Read the model definition and answer for the solid it produces. Units are mm, in the model's axes. Face numbers are marked on the shaded views. Coordinates: 2 decimals unless noted, no trailing zeros. Loops run counter-clockwise (first coordinate to the right, second up) from the corner with the lowest first, then second, coordinate; pieces in that order, holes last. Notation, with made-up numbers: M 45.5,-4.75 L 68.5,-4.75 A35 ccw 68.5,28.25 Z; hole C 41,28.5 d3. An arc over 180 degrees is marked long. One line per item, written item: value. Start each with the question number.
1. The part is cut by section A-A (x = 10). Write down the section's boundary in (y, z), then the cut area to 3 significant figures.
2. Determine the mould class of the marked faces 1, 2, 3 and 4 for opening direction X: +X half, -X half, draft (parallel to the pull), parting line (faces both ways), or undercut.
3. Flat-ended cylindrical pins translate along their axes: pin 1 (3 mm diameter, centred on x = 0, y = -2, fed in from -Z); pin 2 (5 mm diameter, centred on y = 6, z = 1.5, fed in from +X); pin 3 (5 mm diameter, centred on y = -5, z = 1.5, fed in from -X); pin 4 (4.5 mm diameter, centred on x = 10, y = 10, fed in from -Z). Find the tip coordinate at first contact, or state that the pin passes through.
4. Consider probe 1 along X at (y, z) = (10, 9.05); probe 2 along Y at (x, z) = (10, 4.75); probe 3 along Y at (x, z) = (-10, 9.2). Determine where each line is inside the solid, lowest interval first.
5. The part is cut by section B-B (z = 5.5). Write down the section's boundary in (x, y), then the cut area to 3 significant figures.
6. The part is cut by section D-D (y = -2.5). Write down the section's boundary in (x, z), then the cut area to 3 significant figures.
Autodesk Fusion 360 part; units mm, degrees
sketch "Sketch1" plane through (0, 0, 0) normal (0, 0, 1) x (1, 0, 0)
  line L0 (20, -20) -> (-20, -20)
  line L1 (-20, -20) -> (-20, 20)
  line L2 (-20, 20) -> (20, 20)
  line L3 (20, 20) -> (20, -20)
  line L4 (20, -20) -> (-20, 20) construction
  line L5 (-20, -20) -> (20, 20) construction
  dimension "d1" = 40
  dimension "d2" = 40
extrude "Extrude1" add sketch "Sketch1" along normal blind 5
chamfer "Chamfer1" distance 8 angle 30 4 edges at (20, 0, 0) (0, -20, 0) (-20, 0, 0) (0, 20, 0) measured on face at (6.6667, -6.6667, 0) measured on face at (6.6667, -6.6667, 0) measured on face at (6.6667, -6.6667, 0) measured on face at (6.6667, -6.6667, 0)
extrude "Extrude2" add 1 faces at (6.6667, -6.6667, 5) along direction (0, 0, 1) blind 5
sketch "Sketch2" plane through (0, 0, 10) normal (0, 0, 1) x (-1, 0, 0)
  line L0 (-20, -20) -> (20, -20)
  line L1 (20, -20) -> (20, 20)
  line L2 (20, 20) -> (-20, 20)
  line L3 (-20, 20) -> (-20, -20)
  circle A0 centre (10, 10) radius 2.5
  circle A1 centre (-10, -10) radius 2.5
  circle A2 centre (10, 10) radius 4.5
  circle A3 centre (-10, -10) radius 4.5
  dimension "d11" = 5
  dimension "d12" = 5
  dimension "d15" = 9
  dimension "d16" = 9
  dimension "d20" = 10
  dimension "d21" = 10
  dimension "d22" = 10
  dimension "d23" = 10
extrude "Extrude4" cut sketch "Sketch2" along normal blind 7 from surface at -10 contours A2 | A3
extrude "Extrude3" cut sketch "Sketch2" against normal up to surface (10 mm away) contours A0 | A1
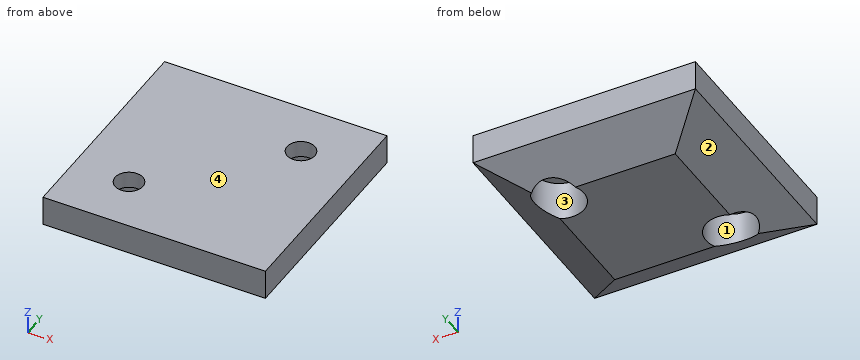
Answer block:
1. outline: M -20,4.62 L -12,0 L 5.5,0 L 5.5,7 L 7.5,7 L 7.5,10 L -20,10 Z; M 12.5,7 L 14.5,7 L 14.5,1.44 L 20,4.62 L 20,10 L 12.5,10 Z
1. area: 287 mm2
2. face 1: undercut
2. face 2: -X half
2. face 3: undercut
2. face 4: draft
3. pin 1: stops at z = 0
3. pin 2: stops at x = 18.93
3. pin 3: stops at x = -18.93
3. pin 4: passes through
4. probe 1: x = -20 to 7.5, 12.5 to 20
4. probe 2: y = -20 to 5.5, 14.5 to 20
4. probe 3: y = -20 to -12.5, -7.5 to 20
5. outline: M -20,-20 L 20,-20 L 20,20 L -20,20 Z; hole C -10,-10 d9; hole C 10,10 d9
5. area: 1,470 mm2
6. outline: M -20,4.62 L -12,0 L 12,0 L 20,4.62 L 20,10 L -20,10 Z
6. area: 363 mm2
